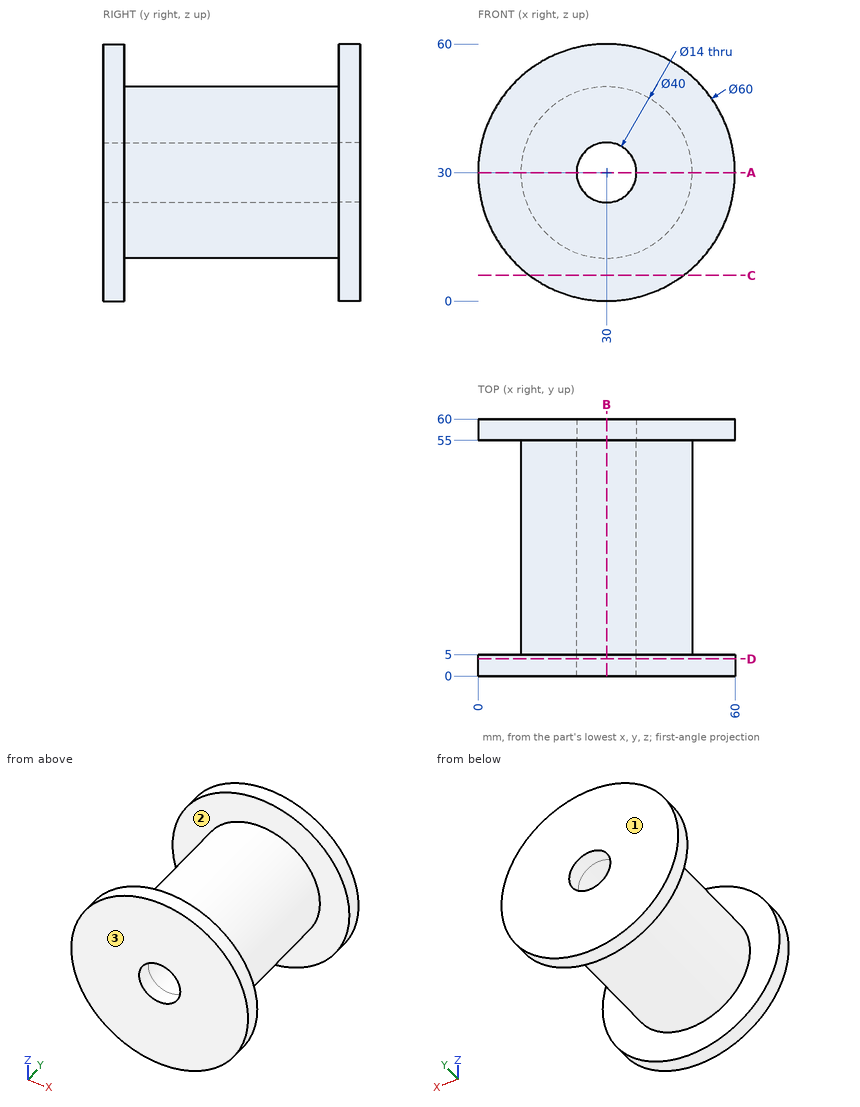
Print and shaded views of the part. All mm, measured from the part's lowest x, y and z. Round coordinates to 2 decimals unless told otherwise and drop trailing zeros. Write each loop counter-clockwise with the first axis right and the second up, starting at its lowest first coordinate (ties: lowest second). Pieces come first, ordered by that corner, then holes. Notation, with made-up numbers: (-7.75, 38.5) -> (9.25, 38.5) arc R23 ccw to (9.25, 72.5) -> close; hole circle Ø10 at (37.25, 79). An arc over 180 degrees is marked (long way). Return JSON: item names as keys, results as strings. Group by question number.
Q1. Saw through at D-D on y = 4. Write the cut outline in (x, z).
Q2. Mould opens along Y. For the marked faces 1, 2 and 3 say: pulls with the +Y half, pulls with the -Y half, needs draft (parallel to the pull), parting line crosses it, or undercut.
Q3. Saw through at C-C on z = 6. Write the cut outline in (x, y), plus the area to 3 significant figures.
Q4. Saw through at B-B on x = 30. Write the cut outline in (y, z).
Q5. Probe L1, parallel to Z at x = 30, y = 34; L2, parallel to Y at x = 51, z = 9; L3, parallel to Z at x = 30, y = 3.7. List the from-to ranges inside material, lowest first. Write a range as [from, to].
Q6. Saw through at A-A on z = 30. Write the cut outline in (x, y).
Q7. Pin check, flat tips, straight feed: pin 1 (1.5 mm diameter, centred on y = 27, z = 25, fed in from +X); pin 2 (6 mm diameter, centred on y = 29.5, z = 10.5, fed in from -X); pin 3 (1 mm diameter, centred on x = 19.5, y = 22.5, fed in from -Z). Stop position of each tip, or through.
Answer:
{
 "1": {"outline": "circle Ø60 at (30, 30); hole circle Ø14 at (30, 30)"},
 "2": {"face 1": "pulls with the +Y half", "face 2": "undercut", "face 3": "pulls with the -Y half"},
 "3": {"outline": "(12, 0) -> (48, 0) -> (48, 5) -> (12, 5) -> close; (12, 55) -> (48, 55) -> (48, 60) -> (12, 60) -> close", "area": "360 mm2"},
 "4": {"outline": "(0, 0) -> (5, 0) -> (5, 10) -> (55, 10) -> (55, 0) -> (60, 0) -> (60, 23) -> (0, 23) -> close; (0, 37) -> (60, 37) -> (60, 60) -> (55, 60) -> (55, 50) -> (5, 50) -> (5, 60) -> (0, 60) -> close"},
 "5": {"L1": "[10, 23], [37, 50]", "L2": "[0, 5], [55, 60]", "L3": "[0, 23], [37, 60]"},
 "6": {"outline": "(0, 0) -> (23, 0) -> (23, 60) -> (0, 60) -> (0, 55) -> (10, 55) -> (10, 5) -> (0, 5) -> close; (37, 0) -> (60, 0) -> (60, 5) -> (50, 5) -> (50, 55) -> (60, 55) -> (60, 60) -> (37, 60) -> close"},
 "7": {"pin 1": "x = 49.54", "pin 2": "x = 18.7", "pin 3": "z = 12.68"}
}
